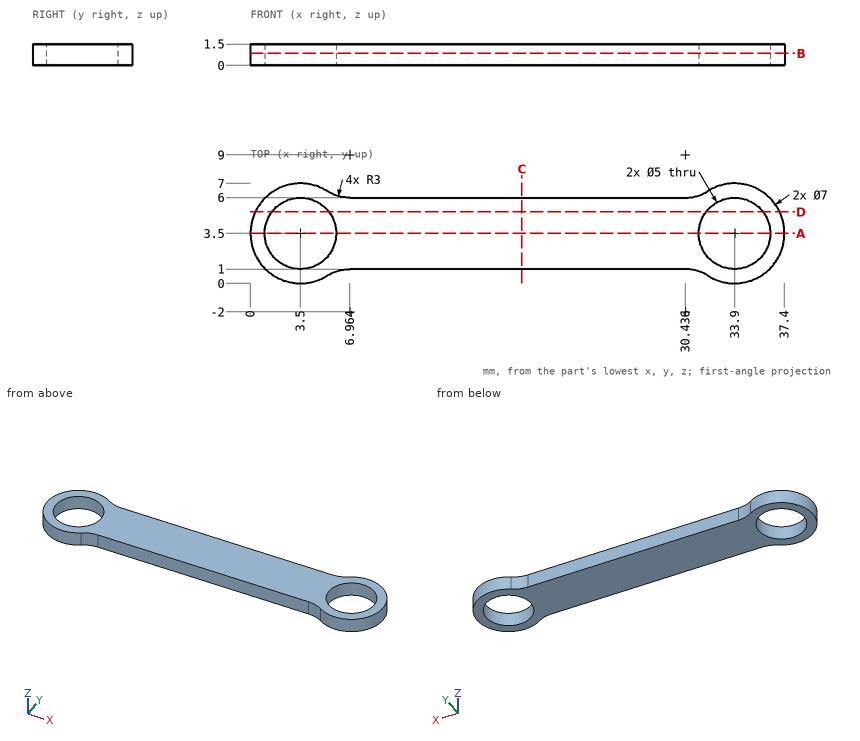
For this review, use the dimensioned drawing (mm, ordinates from the lowest corner) and the shaded views. Give positions to 0.01 mm unless a question says otherwise; leave off trailing zeros. Order: outer loops, then holes, each group sorted by start corner. A loop starts at its lowest first (then second) coordinate and runs counter-clockwise, first axis right, second up.
1. Add section B-B, the plane z = 0.85. State the section outline as (x, y) points, then the cut area to 3 significant figures.
Solution:
outline: (5.37, 0.54) arc R3 cw to (6.96, 1) - (30.44, 1) arc R3 cw to (32.03, 0.54) arc R3.5 ccw (long way) to (32.03, 6.46) arc R3 cw to (30.44, 6) - (6.96, 6) arc R3 cw to (5.37, 6.46) arc R3.5 ccw (long way) to start; hole circle Ø5 at (3.5, 3.5); hole circle Ø5 at (33.9, 3.5)
area: 158 mm2
2. Add section A-A, the plane y = 3.5. State the section outline as (x, z) points.
Solution:
outline: (0, 0) - (1, 0) - (1, 1.5) - (0, 1.5) - close; (6, 0) - (31.4, 0) - (31.4, 1.5) - (6, 1.5) - close; (36.4, 0) - (37.4, 0) - (37.4, 1.5) - (36.4, 1.5) - close
3. To check wall thickness, follow L1, parallel to X at y = 5, z = 0.8; L2, parallel to X at y = 4, z = 1; L3, parallel to Y at x = 19.5, z = 0.4. State the ranges of each line that lie inside material, in increasing order.
Solution:
L1: x = 0.34 to 1.5, 5.5 to 31.9, 35.9 to 37.06
L2: x = 0.04 to 1.05, 5.95 to 31.45, 36.35 to 37.36
L3: y = 1 to 6
4. Add section C-C, the plane x = 19. State the section outline as (y, z) points.
Solution:
outline: (1, 0) - (6, 0) - (6, 1.5) - (1, 1.5) - close
5. Add section D-D, the plane y = 5. State the section outline as (x, z) points.
Solution:
outline: (0.34, 0) - (1.5, 0) - (1.5, 1.5) - (0.34, 1.5) - close; (5.5, 0) - (31.9, 0) - (31.9, 1.5) - (5.5, 1.5) - close; (35.9, 0) - (37.06, 0) - (37.06, 1.5) - (35.9, 1.5) - close
